Study the drawing (mm; zero at the part's minimum x, y, z) and answer. A direction names the side the tool comes from. Round coordinates to 2 decimals unless told otherwise and drop trailing zeros. Write each loop counter-clockwise with the first axis right and the second up, starting at its lowest first coordinate (ties: lowest second). Pieces come first, ordered by that corner, then holes.
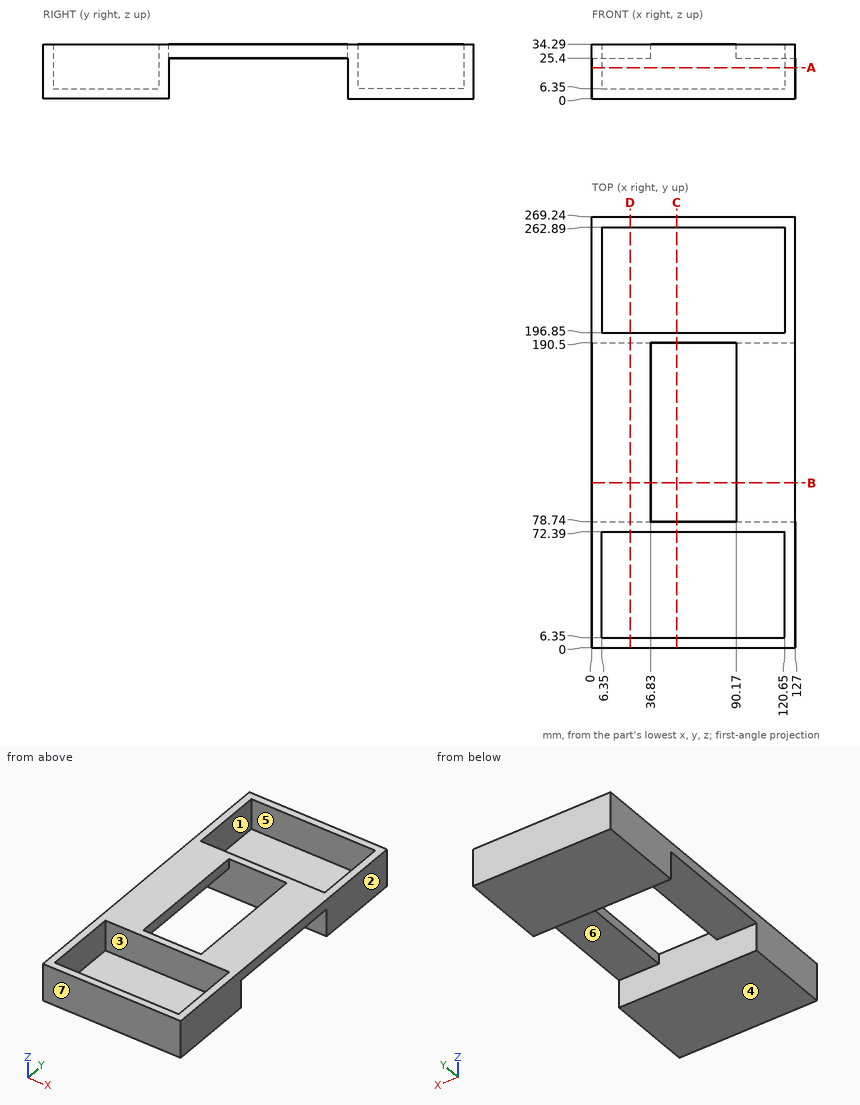
1. Given pin 1 (20 mm diameter, centred on x = 50, y = 244.5, fed in from +Z), flat-ended and moving along its own axis, determine where the tip first touches the part or whether it passes through.
Geometry says:
pin 1: stops at z = 6.35
2. Section C-C on x = 53 is taken. Determine the outline of the cut face in (y, z).
Geometry says:
outline: (0, 0) - (78.74, 0) - (78.74, 34.29) - (72.39, 34.29) - (72.39, 6.35) - (6.35, 6.35) - (6.35, 34.29) - (0, 34.29) - close; (190.5, 0) - (269.24, 0) - (269.24, 34.29) - (262.89, 34.29) - (262.89, 6.35) - (196.85, 6.35) - (196.85, 34.29) - (190.5, 34.29) - close
3. Section B-B on y = 103 is taken. Determine the outline of the cut face in (x, z).
Geometry says:
outline: (0, 25.4) - (36.83, 25.4) - (36.83, 34.29) - (0, 34.29) - close; (90.17, 25.4) - (127, 25.4) - (127, 34.29) - (90.17, 34.29) - close
4. Section A-A on z = 19.5 is taken. Determine the outline of the cut face in (x, y).
Geometry says:
outline: (0, 0) - (127, 0) - (127, 78.74) - (0, 78.74) - close; (0, 190.5) - (127, 190.5) - (127, 269.24) - (0, 269.24) - close; hole (6.35, 6.35) - (120.65, 6.35) - (120.65, 72.39) - (6.35, 72.39) - close; hole (6.35, 196.85) - (120.65, 196.85) - (120.65, 262.89) - (6.35, 262.89) - close
5. A tool of negligible diameter and unlimited length cuts with its end or side. For the marked faces 5, 6 and 7, from which of +Z, -Z, +X, -X, +Y, -Y can it reach the whole face along a straight path? Write none if from no direction.
Geometry says:
face 5: +Z
face 6: -Z, +X, -X
face 7: +Z, -Z, +X, -X, -Y
6. Straight lines are drawn through the part: line 1 along Y through (x, z) = (53.5, 8); line 2 along Y through (x, z) = (24, 28); line 3 along X through (y, z) = (215, 19). For each, find the intervals that lie inside material, in ascending order.
Geometry says:
line 1: y = 0 to 6.35, 72.39 to 78.74, 190.5 to 196.85, 262.89 to 269.24
line 2: y = 0 to 6.35, 72.39 to 196.85, 262.89 to 269.24
line 3: x = 0 to 6.35, 120.65 to 127
7. For a pull along X with two mould halves and no side action, classify the marked faces 1, 2, 3 and 4 as released by +X, released by -X, zero draft, split by the parting line, or undercut.
Geometry says:
face 1: undercut
face 2: released by +X
face 3: undercut
face 4: zero draft
8. Section D-D on x = 24 is taken. Determine the outline of the cut face in (y, z), plus the area to 3 significant figures.
Geometry says:
outline: (0, 0) - (78.74, 0) - (78.74, 25.4) - (190.5, 25.4) - (190.5, 0) - (269.24, 0) - (269.24, 34.29) - (262.89, 34.29) - (262.89, 6.35) - (196.85, 6.35) - (196.85, 34.29) - (72.39, 34.29) - (72.39, 6.35) - (6.35, 6.35) - (6.35, 34.29) - (0, 34.29) - close
area: 2,700 mm2
